```python
from build123d import *

# Parameters (mm, degrees)
BOSS_EXTRUDE1_DEPTH                       = 33.5
BOSS_EXTRUDE2_DEPTH                       = 21.25
FILLET3_R                                 = 5
CUT_EXTRUDE3_REACH                        = 106.891
SKETCH14_W                                = 2.5
SKETCH14_H                                = 40
M2X0_4_TAPPED_HOLE1_D                     = 1.6
TAPPED_HOLE_FOR_M2_5X0_45_HELICOIL1_D     = 2.55
TAPPED_HOLE_FOR_M2_5X0_45_HELICOIL1_DEPTH = 4.5
TAPPED_HOLE_FOR_M2_5X0_45_HELICOIL1_TIP   = 0.766097289
SKETCH22_W                                = 29
SKETCH22_H                                = 7
CUT_EXTRUDE4_DEPTH                        = 21.58
FILLET5_R                                 = 2.5
SKETCH23_W                                = 12.652347045
SKETCH23_H                                = 3.5
SKETCH23_W_2                              = 11.018435539
CUT_EXTRUDE5_DEPTH                        = 2


with BuildPart() as part:
    # Sketch1 → Boss-Extrude1 (new, symmetric)
    with BuildSketch(Plane.XY):
        with BuildLine():
            Line((0, 0), (4.5, 0))
            Line((4.5, 0), (4.5, -10))
            ThreePointArc((4.5, -10), (11.761387212, -19.617692031), (23, -15.267826876))
            Line((23, -15.267826876), (25, -15.267826876))
            ThreePointArc((25, -15.267826876), (36.238612788, -19.617692031), (43.5, -10))
            Line((43.5, -10), (46.1, -10))
            ThreePointArc((46.1, -10), (53.361387212, -19.617692031), (64.6, -15.267826876))
            Line((64.6, -15.267826876), (66.6, -15.267826876))
            ThreePointArc((66.6, -15.267826876), (77.838612788, -19.617692031), (85.1, -10))
            Line((85.1, -10), (85.1, 0))
            Line((85.1, 0), (89.6, 0))
            Line((89.6, 0), (89.6, -4.5))
            Line((89.6, -4.5), (87.1, -4.5))
            Line((87.1, -4.5), (87.1, -10))
            ThreePointArc((87.1, -10), (83.585281374, -18.485281374), (75.1, -22))
            Line((75.1, -22), (14.5, -22))
            ThreePointArc((14.5, -22), (6.014718626, -18.485281374), (2.5, -10))
            Line((2.5, -10), (2.5, -4.5))
            Line((2.5, -4.5), (0, -4.5))
            Line((0, -4.5), (0, 0))
        make_face()
    extrude(amount=BOSS_EXTRUDE1_DEPTH, both=True)

    # Sketch9 → Boss-Extrude2 (add, symmetric)
    with BuildSketch(Plane.ZY.offset(-44.8)):
        Polygon((33.5, -22), (38.5, -22), (38.5, 0), (49.9, 0), (49.9, 1.58), (33.5, 1.58), align=None)
    boss_extrude2 = extrude(amount=BOSS_EXTRUDE2_DEPTH, both=True)

    # Mirror1: Boss-Extrude2 across plane
    add(boss_extrude2.mirror(Plane.XY))

    # Fillet3
    fillet3_edges = [part.edges().sort_by_distance(p)[0] for p in [
        (44.8, -22, -38.5),
        (44.8, 0, -38.5),
        (44.8, 0, 38.5),
        (44.8, -22, 38.5),
    ]]
    fillet(fillet3_edges, radius=FILLET3_R)

    # Sketch14 → Cut-Extrude3 (cut, up to next)
    with BuildSketch(Plane(origin=(0, 0, 0), x_dir=(1, 0, 0), z_dir=(0, 1, 0)), mode=Mode.PRIVATE) as cut_extrude3_sk1:
        with Locations((1.25, 0)):
            Rectangle(SKETCH14_W, SKETCH14_H)
    cut_extrude3_tool1 = extrude(cut_extrude3_sk1.sketch, amount=-CUT_EXTRUDE3_REACH, mode=Mode.PRIVATE) & part.part
    add(cut_extrude3_tool1.solids().sort_by_distance((1.25, 0, 0))[0], mode=Mode.SUBTRACT)

    # M2x0.4 Tapped Hole1 (through all)
    with Locations(Plane(origin=(0, -10, 0), x_dir=(1, 0, 0), z_dir=(0, 1, 0))):
        with Locations((44.8, 15), (44.8, -15)):
            Hole(M2X0_4_TAPPED_HOLE1_D / 2)

    # Tapped Hole for M2.5x0.45 Helicoil1
    with Locations(Plane(origin=(0, 0, 0), x_dir=(1, 0, 0), z_dir=(0, 1, 0))):
        with Locations((2.25, 25), (2.25, -25), (87.35, -25), (87.35, 25)):
            Hole(TAPPED_HOLE_FOR_M2_5X0_45_HELICOIL1_D / 2, depth=TAPPED_HOLE_FOR_M2_5X0_45_HELICOIL1_DEPTH)
            with Locations((0, 0, -(TAPPED_HOLE_FOR_M2_5X0_45_HELICOIL1_DEPTH + TAPPED_HOLE_FOR_M2_5X0_45_HELICOIL1_TIP / 2))):  # 118° drill point
                Cone(0, TAPPED_HOLE_FOR_M2_5X0_45_HELICOIL1_D / 2, TAPPED_HOLE_FOR_M2_5X0_45_HELICOIL1_TIP, mode=Mode.SUBTRACT)

    # Sketch22 → Cut-Extrude4 (cut)
    with BuildSketch(Plane(origin=(0, 1.58, 0), x_dir=(1, 0, 0), z_dir=(0, 1, 0))):
        with Locations((29, 30)):
            Rectangle(SKETCH22_W, SKETCH22_H)
        with Locations((60.6, 30)):
            Rectangle(SKETCH22_W, SKETCH22_H)
        with Locations((29, -30)):
            Rectangle(SKETCH22_W, SKETCH22_H)
        with Locations((60.6, -30)):
            Rectangle(SKETCH22_W, SKETCH22_H)
    extrude(amount=-CUT_EXTRUDE4_DEPTH, mode=Mode.SUBTRACT)

    # Fillet5
    # the kernel refuses this fillet: 2.5 mm, written as the material it adds along each edge
    with BuildSketch(Plane(origin=(23.55, -20, -33.5), x_dir=(0, 0, -1), z_dir=(0, -1, 0))) as fillet5_piece_1_section:
        with BuildLine():
            CenterArc((FILLET5_R, -FILLET5_R), FILLET5_R, 90, 90)
            Line((0, -FILLET5_R), (0, 0))
            Line((0, 0), (FILLET5_R, 0))
        make_face()
    fillet5_piece_1 = extrude(amount=8.25, mode=Mode.PRIVATE)
    fillet5_piece_1 = fillet5_piece_1 & Plane(origin=(22.982039754, -17, -33.5), x_dir=(0, -1, 0), z_dir=(-1, 0, 0)) * Cylinder(5, 27, mode=Mode.PRIVATE)
    add(fillet5_piece_1)
    with BuildSketch(Plane(origin=(66.05, -20, -33.5), x_dir=(0, 0, -1), z_dir=(0, -1, 0))) as fillet5_piece_2_section:
        with BuildLine():
            CenterArc((FILLET5_R, FILLET5_R), FILLET5_R, 180, 90)
            Line((0, FILLET5_R), (0, 0))
            Line((0, 0), (FILLET5_R, 0))
        make_face()
    fillet5_piece_2 = extrude(amount=8.25, mode=Mode.PRIVATE)
    fillet5_piece_2 = fillet5_piece_2 & Plane(origin=(66.617960246, -17, -33.5), x_dir=(0, -1, 0), z_dir=(-1, 0, 0)) * Cylinder(5, 27, mode=Mode.PRIVATE)
    add(fillet5_piece_2)
    with BuildSketch(Plane(origin=(66.05, -20, 33.5), x_dir=(0, 0, 1), z_dir=(0, -1, 0))) as fillet5_piece_3_section:
        with BuildLine():
            CenterArc((FILLET5_R, -FILLET5_R), FILLET5_R, 90, 90)
            Line((0, -FILLET5_R), (0, 0))
            Line((0, 0), (FILLET5_R, 0))
        make_face()
    fillet5_piece_3 = extrude(amount=8.25, mode=Mode.PRIVATE)
    fillet5_piece_3 = fillet5_piece_3 & Plane(origin=(66.617960246, -17, 33.5), x_dir=(0, -1, 0), z_dir=(-1, 0, 0)) * Cylinder(5, 27, mode=Mode.PRIVATE)
    add(fillet5_piece_3)
    with BuildSketch(Plane(origin=(23.55, -20, 33.5), x_dir=(0, 0, 1), z_dir=(0, -1, 0))) as fillet5_piece_4_section:
        with BuildLine():
            CenterArc((FILLET5_R, FILLET5_R), FILLET5_R, 180, 90)
            Line((0, FILLET5_R), (0, 0))
            Line((0, 0), (FILLET5_R, 0))
        make_face()
    fillet5_piece_4 = extrude(amount=8.25, mode=Mode.PRIVATE)
    fillet5_piece_4 = fillet5_piece_4 & Plane(origin=(22.982039754, -17, 33.5), x_dir=(0, -1, 0), z_dir=(-1, 0, 0)) * Cylinder(5, 27, mode=Mode.PRIVATE)
    add(fillet5_piece_4)
    with BuildSketch(Plane(origin=(2.5, 0, 20), x_dir=(-1, 0, 0), z_dir=(0, -1, 0)), Plane(origin=(2.5, 0, -20), x_dir=(0, 0, 1), z_dir=(0, -1, 0))) as fillet5_piece_5:
        with BuildLine():
            CenterArc((FILLET5_R, FILLET5_R), FILLET5_R, 180, 90)
            Line((0, FILLET5_R), (0, 0))
            Line((0, 0), (FILLET5_R, 0))
        make_face()
    extrude(amount=4.5)
    with BuildSketch(Plane(origin=(43.5, -10, -26.5), x_dir=(-1, 0, 0), z_dir=(0, -1, 0))) as fillet5_piece_6_section:
        with BuildLine():
            CenterArc((FILLET5_R, FILLET5_R), FILLET5_R, 180, 90)
            Line((0, FILLET5_R), (0, 0))
            Line((0, 0), (FILLET5_R, 0))
        make_face()
    fillet5_piece_6 = extrude(amount=10, mode=Mode.PRIVATE)
    fillet5_piece_6 = fillet5_piece_6 - Plane(origin=(33.5, -10, -27.115850249), x_dir=(-0.8499999999999996, -0.5267826876426376, 0), z_dir=(0, 0, 1)) * Cylinder(10, 30, mode=Mode.PRIVATE)
    add(fillet5_piece_6)
    with BuildSketch(Plane(origin=(43.5, -10, -33.5), x_dir=(0, 0, 1), z_dir=(0, -1, 0)), Plane(origin=(43.5, -10, 33.5), x_dir=(-1, 0, 0), z_dir=(0, -1, 0))) as fillet5_piece_7:
        with BuildLine():
            CenterArc((FILLET5_R, FILLET5_R), FILLET5_R, 180, 90)
            Line((0, FILLET5_R), (0, 0))
            Line((0, 0), (FILLET5_R, 0))
        make_face()
    extrude(amount=10)
    with BuildSketch(Plane(origin=(43.5, -10, 26.5), x_dir=(-1, 0, 0), z_dir=(0, -1, 0))) as fillet5_piece_8_section:
        with BuildLine():
            CenterArc((FILLET5_R, -FILLET5_R), FILLET5_R, 90, 90)
            Line((0, -FILLET5_R), (0, 0))
            Line((0, 0), (FILLET5_R, 0))
        make_face()
    fillet5_piece_8 = extrude(amount=10, mode=Mode.PRIVATE)
    fillet5_piece_8 = fillet5_piece_8 - Plane(origin=(33.5, -10, 27.115850249), x_dir=(-0.8499999999999996, -0.5267826876426376, 0), z_dir=(0, 0, 1)) * Cylinder(10, 30, mode=Mode.PRIVATE)
    add(fillet5_piece_8)
    with BuildSketch(Plane(origin=(46.1, -10, 33.5), x_dir=(1, 0, 0), z_dir=(0, -1, 0)), Plane(origin=(46.1, -10, -33.5), x_dir=(0, 0, 1), z_dir=(0, -1, 0))) as fillet5_piece_9:
        with BuildLine():
            CenterArc((FILLET5_R, -FILLET5_R), FILLET5_R, 90, 90)
            Line((0, -FILLET5_R), (0, 0))
            Line((0, 0), (FILLET5_R, 0))
        make_face()
    extrude(amount=10)
    with BuildSketch(Plane(origin=(46.1, -10, 26.5), x_dir=(1, 0, 0), z_dir=(0, -1, 0))) as fillet5_piece_10_section:
        with BuildLine():
            CenterArc((FILLET5_R, FILLET5_R), FILLET5_R, 180, 90)
            Line((0, FILLET5_R), (0, 0))
            Line((0, 0), (FILLET5_R, 0))
        make_face()
    fillet5_piece_10 = extrude(amount=10, mode=Mode.PRIVATE)
    fillet5_piece_10 = fillet5_piece_10 - Plane(origin=(56.1, -10, 27.115850543), x_dir=(-1, 0, 0), z_dir=(0, 0, 1)) * Cylinder(10, 30, mode=Mode.PRIVATE)
    add(fillet5_piece_10)
    with BuildSketch(Plane(origin=(46.1, -10, -26.5), x_dir=(1, 0, 0), z_dir=(0, -1, 0))) as fillet5_piece_11_section:
        with BuildLine():
            CenterArc((FILLET5_R, -FILLET5_R), FILLET5_R, 90, 90)
            Line((0, -FILLET5_R), (0, 0))
            Line((0, 0), (FILLET5_R, 0))
        make_face()
    fillet5_piece_11 = extrude(amount=10, mode=Mode.PRIVATE)
    fillet5_piece_11 = fillet5_piece_11 - Plane(origin=(56.1, -10, -27.115850543), x_dir=(-1, 0, 0), z_dir=(0, 0, 1)) * Cylinder(10, 30, mode=Mode.PRIVATE)
    add(fillet5_piece_11)

    # Sketch23 → Cut-Extrude5 (cut)
    with BuildSketch(Plane(origin=(0, -10, 0), x_dir=(1, 0, 0), z_dir=(0, 1, 0))):
        with Locations((44.873232105, 15)):
            Rectangle(SKETCH23_W, SKETCH23_H)
        with Locations((44.351234715, -15)):
            Rectangle(SKETCH23_W_2, SKETCH23_H)
    extrude(amount=-CUT_EXTRUDE5_DEPTH, mode=Mode.SUBTRACT)


solid = part.part
```
Here's how the part is built. I have some questions about the finished solid (model axes, mm). A direction names the side the tool comes from. Coordinates: 2 decimals unless noted, no trailing zeros. Loops run counter-clockwise (first coordinate to the right, second up) from the corner with the lowest first, then second, coordinate; pieces in that order, holes last. Notation, with made-up numbers: M 77.5,9 L 136.5,9 A22 ccw 136.5,39 Z; hole C 52,14 d8. An arc over 180 degrees is marked long. One line per item, written item: value.
1. On a 3-axis mill with a long thin cutter (end or side, diameter ignored), from which of +Z, -Z, +X, -X, +Y, -Y can I reach the whole of each face in a straight line? I mean faces 1 (the flat face through (85.1, -5, 0)), 2 (the flat face through (45, -9, 33.5)), 3 (the flat face through (23.55, -7, 38)), 4 (the flat face through (45, -11, -38.5)). Say none if no direction works.
Geometry says:
face 1: +Z, -Z, +Y
face 2: +Y
face 3: +Z, -X, +Y
face 4: -Z, +X, -X, -Y
2. Thinking about a two-plate mould opening in X: for faces 5 (the flat face through (1, -4.5, -27)), 6 (the cylindrical face through (22.798, -20.986, 34.213)), 7 (the flat face through (45, -12, -16)), which applies, +X half, -X half, draft (parallel to the pull), parting line (faces both ways), or undercut?
Geometry says:
face 5: draft
face 6: -X half
face 7: undercut
3. Imagine slicing it at C-C (y = -18.5). State how many separate pieces and enclosed holes the cut face has, and give its area (3 significant figures).
Geometry says:
separate pieces: 5
enclosed holes: 2
area: 2,410 mm2
4. Will these pins go through, and if not, where does the flat tip stop? pin 1 Ø1.9 at (x, z) = (39.5, -45) entering from -Y; pin 2 Ø1.6 at (y, z) = (-6.5, -16.5) entering from +X; pin 3 Ø1 at (x, z) = (24, 3) entering from +Y; pin 4 Ø5 at (x, z) = (23, 32.5) entering from +Y.
Geometry says:
pin 1: stops at y = 0
pin 2: stops at x = 87.1
pin 3: stops at y = -15.27
pin 4: stops at y = 1.58
5. Imagine slicing it at B-B (z = -10). List the corners of the cut face in (x, y) for me, and give its area (3 significant figures).
Geometry says:
outline: M 2.5,-10 A12 ccw 14.5,-22 L 75.1,-22 A12 ccw 87.1,-10 L 87.1,-4.5 L 89.6,-4.5 L 89.6,0 L 85.1,0 L 85.1,-10 A10 cw 66.6,-15.27 L 64.6,-15.27 A10 cw 46.1,-10 L 43.5,-10 A10 cw 25,-15.27 L 23,-15.27 A10 cw 4.5,-10 L 4.5,0 L 2.5,0 Z
area: 377 mm2
6. Please list where these lines run through material, in increasing order: probe 1 along Z at (x, y) = (87.35, -1.95) (3 decimals); probe 2 along X at (y, z) = (-0.95, -25) (3 decimals); probe 3 along Z at (x, y) = (44.8, -16.75).
Geometry says:
probe 1: z = -33.5 to -26.275, -23.725 to 23.725, 26.275 to 33.5
probe 2: x = 0 to 0.975, 3.525 to 4.5, 85.1 to 86.075, 88.625 to 89.6
probe 3: z = -38.5 to -15.8, -14.2 to 14.2, 15.8 to 38.5
7. Imagine slicing it at A-A (z = 25). List the corners of the cut face in (x, y) for me (3 decimals).
Geometry says:
outline: M 0,-4.5 L 0.975,-4.5 L 0.975,0 L 0,0 Z; M 2.5,-10 A12 ccw 14.5,-22 L 75.1,-22 A12 ccw 87.1,-10 L 87.1,-5.116 L 86.075,-4.5 L 86.075,0 L 85.1,0 L 85.1,-10 A10 cw 66.6,-15.268 L 64.6,-15.268 A10 cw 46.1,-10 L 43.5,-10 A10 cw 25,-15.268 L 23,-15.268 A10 cw 4.5,-10 L 4.5,0 L 3.525,0 L 3.525,-4.5 L 2.5,-5.116 Z; M 88.625,-4.5 L 89.6,-4.5 L 89.6,0 L 88.625,0 Z
8. Imagine slicing it at D-D (x = 28). List the corners of the cut face in (y, z) for me.
Geometry says:
outline: M -22,-33.5 A5 ccw -17,-38.5 L -5,-38.5 A5 cw 0,-43.5 L 0,-49.9 L 1.58,-49.9 L 1.58,-33.5 L -20,-33.5 L -20,-26.5 L -18.35,-26.5 L -18.35,26.5 L -20,26.5 L -20,33.5 L 1.58,33.5 L 1.58,49.9 L 0,49.9 L 0,43.5 A5 cw -5,38.5 L -17,38.5 A5 ccw -22,33.5 Z
